```python
from build123d import *

# Parameters (mm, degrees)
BOSS_EXTRUDE1_DEPTH                            = 21
CBORE_FOR_6_SOCKET_HEAD_CAP_SCREW1_D           = 3.6576
CBORE_FOR_6_SOCKET_HEAD_CAP_SCREW1_DEPTH       = 9.398
CBORE_FOR_6_SOCKET_HEAD_CAP_SCREW1_CBORE_D     = 7.14502
CBORE_FOR_6_SOCKET_HEAD_CAP_SCREW1_CBORE_DEPTH = 2.54
CBORE_FOR_6_SOCKET_HEAD_CAP_SCREW1_TIP         = 1.0988539
F_6_CLEARANCE_HOLE1_D                          = 3.6576
FILLET1_R                                      = 0.75
SKETCH8_W                                      = 4
SKETCH8_H                                      = 10.668
CUT_EXTRUDE1_DEPTH                             = 7.3500001


with BuildPart() as part:
    # Sketch1 → Boss-Extrude1 (new body, symmetric)
    with BuildSketch(Plane(origin=(0, 0, 0), x_dir=(0, 0, -1), z_dir=(1, 0, 0))):
        Polygon((0, 6.35), (3.175, 9.525), (6.35, 9.525), (6.35, -9.525), (0, -9.525), align=None)
    extrude(amount=BOSS_EXTRUDE1_DEPTH, both=True)

    # CBORE for #6 Socket Head Cap Screw1
    with Locations(Plane(origin=(0, 0, -6.35), x_dir=(-1, 0, 0), z_dir=(0, 0, -1))):
        with Locations((11.525, -5.025), (-11.525, 5.025), (-11.525, -5.025), (11.525, 5.025)):
            CounterBoreHole(CBORE_FOR_6_SOCKET_HEAD_CAP_SCREW1_D / 2, CBORE_FOR_6_SOCKET_HEAD_CAP_SCREW1_CBORE_D / 2, CBORE_FOR_6_SOCKET_HEAD_CAP_SCREW1_CBORE_DEPTH, depth=CBORE_FOR_6_SOCKET_HEAD_CAP_SCREW1_DEPTH)
            with Locations((0, 0, -(CBORE_FOR_6_SOCKET_HEAD_CAP_SCREW1_DEPTH + CBORE_FOR_6_SOCKET_HEAD_CAP_SCREW1_TIP / 2))):  # 118° drill point
                Cone(0, CBORE_FOR_6_SOCKET_HEAD_CAP_SCREW1_D / 2, CBORE_FOR_6_SOCKET_HEAD_CAP_SCREW1_TIP, mode=Mode.SUBTRACT)

    # #6 Clearance Hole1 (through all)
    with Locations(Plane(origin=(0, -9.525, 0), x_dir=(-1, 0, 0), z_dir=(0, -1, 0))):
        with Locations((-15.525, 0), (15.525, 0)):
            Hole(F_6_CLEARANCE_HOLE1_D / 2)

    # Fillet1
    fillet1_edges = [part.edges().sort_by_distance(p)[0] for p in [
        (0, 6.35, 0),
        (0, -9.525, 0),
    ]]
    fillet(fillet1_edges, radius=FILLET1_R)

    # Sketch8 → Cut-Extrude1 (cut, through all)
    with BuildSketch(Plane(origin=(0, 0, -6.35), x_dir=(-1, 0, 0), z_dir=(0, 0, -1))):
        with Locations((-19, 4.191)):
            Rectangle(SKETCH8_W, SKETCH8_H)
    extrude(amount=-CUT_EXTRUDE1_DEPTH, mode=Mode.SUBTRACT)


solid = part.part
```
Check sheet for the modelled part. Datum: model origin and axes. Units: mm. A direction names the side the tool comes from. Give positions to 0.01 mm unless a question says otherwise; leave off trailing zeros. Loops run counter-clockwise (first coordinate to the right, second up) from the corner with the lowest first, then second, coordinate; pieces in that order, holes last. Notation, with made-up numbers: M 2.5,21.25 L 49.5,21.25 A9 ccw 49.5,36.25 Z; hole C 31.25,-16.75 d8. An arc over 180 degrees is marked long. Answer in a Markdown table with one row per item.
1) Cross-section at D-D (y = -7.5). Enter the section's corners in (x, z) (3 decimals), plus the area to 3 significant figures.
Solutions:
| item | result |
|---|---|
| outline | M -21,-6.35 L -14.101,-6.35 L -14.101,-3.81 L -8.949,-3.81 L -8.949,-6.35 L 8.949,-6.35 L 8.949,-3.81 L 14.101,-3.81 L 14.101,-6.35 L 21,-6.35 L 21,0 L 17.354,0 A1.829 cw 13.696,0 L -13.696,0 A1.829 cw -17.354,0 L -21,0 Z |
| area | 230 mm^2 |
2) Mould release check, pull along Y, two halves, no side actions. Record for faces 4 (the face through (14.16, 7.44, -5.1)), 5 (the face through (21, -5, -3)), 6 (the face through (0, -9.525, -3)): released by +Y, released by -Y, zero draft, split by the parting line, or undercut.
Solutions:
| item | result |
|---|---|
| face 4 | undercut |
| face 5 | zero draft |
| face 6 | released by -Y |
3) Thickness scan on line 1 (Y direction, x = 11, z = -3) (3 decimals); line 2 (Y direction, x = 10, z = -5.5) (3 decimals); line 3 (X direction, y = -5.5, z = -6). Record the ranges inside material, lowest first.
Solutions:
| item | result |
|---|---|
| line 1 | y = -9.525 to -6.777, -3.273 to 3.273, 6.777 to 9.35 |
| line 2 | y = -9.525 to -8.256, -1.794 to 1.794, 8.256 to 9.525 |
| line 3 | x = -21 to -15.07, -7.98 to 7.98, 15.07 to 21 |
4) Cross-section at C-C (z = -5). Enter the section's corners in (x, y) (1 decimal), plus the area to 3 significant figures.
Solutions:
| item | result |
|---|---|
| outline | M -21,-9.5 L 21,-9.5 L 21,-1.1 L 17,-1.1 L 17,9.5 L -21,9.5 Z; hole C -11.5,-5 d7.1; hole C -11.5,5 d7.1; hole C 11.5,-5 d7.1; hole C 11.5,5 d7.1 |
| area | 597 mm^2 |
5) Depth check by flat-ended pin: pin 1 (4.5 mm diameter, centred on x = 11.525, y = -5.025, fed in from -Z); pin 2 (6 mm diameter, centred on x = 13.5, y = 4.5, fed in from -Z); pin 3 (2 mm diameter, centred on x = 11.525, y = 5.025, fed in from -Z); pin 4 (1 mm diameter, centred on y = 5.5, z = -2.5, fed in from +X). Enter the tip coordinate at first touch or a pass-through.
Solutions:
| item | result |
|---|---|
| pin 1 | stops at z = -3.81 |
| pin 2 | stops at z = -6.35 |
| pin 3 | passes through |
| pin 4 | stops at x = 17 |
6) Tool access check on faces 1 (the face through (-21, 0, -3)), 2 (the face through (-11.06, 8.567, -5.098)), 3 (the face through (17, 4, -4)). Record the directions out of +Z, -Z, +X, -X, +Y, -Y that give a thin tool (end or side, any length) a straight path to the whole face; none if there is none.
Solutions:
| item | result |
|---|---|
| face 1 | +Z, -Z, -X, +Y, -Y |
| face 2 | -Z |
| face 3 | +Z, -Z, +X, +Y |
7) Cross-section at B-B (y = -5.5). Enter the section's corners in (x, z) (3 decimals), plus the area to 3 significant figures.
Solutions:
| item | result |
|---|---|
| outline | M -21,-6.35 L -15.066,-6.35 L -15.066,-3.81 L -13.291,-3.81 L -13.291,0 L -13.696,0 A1.829 cw -17.354,0 L -21,0 Z; M -9.759,-3.81 L -7.984,-3.81 L -7.984,-6.35 L 7.984,-6.35 L 7.984,-3.81 L 9.759,-3.81 L 9.759,0 L -9.759,0 Z; M 13.291,-3.81 L 15.066,-3.81 L 15.066,-6.35 L 21,-6.35 L 21,0 L 17.354,0 A1.829 cw 13.696,0 L 13.291,0 Z |
| area | 193 mm^2 |
8) Cross-section at A-A (x = -2). Enter the section's corners in (y, z) (3 decimals).
Solutions:
| item | result |
|---|---|
| outline | M -9.525,-6.35 L 9.525,-6.35 L 9.525,-3.175 L 6.57,-0.22 A0.75 ccw 6.039,0 L -8.775,0 A0.75 ccw -9.525,-0.75 Z |
